Autodesk Inventor part; units mm, degrees
ref_plane "YZ Plane" through (0, 0, 0) normal (1, 0, 0) x (0, 1, 0)
ref_plane "XZ Plane" through (0, 0, 0) normal (0, 1, 0) x (-1, 0, 0)
ref_plane "XY Plane" through (0, 0, 0) normal (0, 0, 1) x (1, 0, 0)
sketch "Sketch1" plane through (0, 0, 0) normal (0, 0, 1) x (1, 0, 0)
  line L0 (0, 0) -> (93.5, 0)
  line L1 (93.5, 0) -> (93.5, 150)
  line L2 (93.5, 150) -> (0, 150)
  line L3 (0, 150) -> (0, 0)
  dimension "d0" = 93.5
  dimension "d1" = 150
sketch "Sketch2" plane through (0, 0, 0) normal (1, 0, 0) x (0, 1, 0)
  circle A0 centre (0, 0) radius 12.5
  circle A1 centre (0, 0) radius 8.5
  line L0 (-12.5, 0) -> (12.5, 0)
  line L1 (12.5, 0) -> (12.5, 12.5)
  line L2 (12.5, 12.5) -> (-12.5, 12.5)
  line L3 (-12.5, 12.5) -> (-12.5, 0)
  circle A2 centre (150, 0) radius 12.5
  circle A3 centre (150, 0) radius 8.5
  line L4 (137.5, 0) -> (162.5, 0)
  line L5 (162.5, 0) -> (162.5, 12.5)
  line L6 (162.5, 12.5) -> (137.5, 12.5)
  line L7 (137.5, 12.5) -> (137.5, 0)
  line L8 (-12.5, 12.5) -> (-17.5, 12.5)
  line L9 (-17.5, 12.5) -> (-17.5, 0)
  line L10 (-17.5, 0) -> (-12.5, 0)
  line L11 (-12.5, 0) -> (-12.5, 12.5)
  line L12 (12.5, 12.5) -> (17.5, 12.5)
  line L13 (17.5, 12.5) -> (17.5, 0)
  line L14 (17.5, 0) -> (12.5, 0)
  line L15 (12.5, 0) -> (12.5, 12.5)
  point P0 (8.5, 0)
  point P1 (-8.5, 0)
  point P2 (150, 0)
  point P3 (12.5, 0)
  dimension "d2" = 25
  dimension "d3" = 17
  dimension "d6" = 5
  dimension "d7" = 5
  dimension "d8" = 35
extrude "Extrusion1" add sketch "Sketch2" along normal up to surface (93.5 mm away) contours L3 L2 A0 | A0 L0 A1 | L10 L9 L8 L3 | A0 L2 L1 | L1 L12 L13 L14 | A1 L0 picked at (11.0622, 0.9272) picked at (2.1208, 1.8788)
ref_plane "Work Plane1" through (46.75, 0, 0) normal (-1, 0, 0) x (0, 0, 1)
sketch "Sketch3" plane through (0, -17.5, 0) normal (0, -1, 0) x (1, 0, 0)
  line L0 (0, 12.5) -> (93.5, 12.5)
  line L1 (76, 12.5) -> (111, 12.5)
  line L2 (111, 12.5) -> (111, 0)
  line L3 (111, 0) -> (76, 0)
  line L4 (76, 0) -> (76, 12.5)
  line L5 (93.5, 12.5) -> (93.5, 0)
  circle A0 centre (93.5, 0) radius 8.5
  point P0 (0, 0)
  point P1 (93.5, 12.5)
  point P2 (102, 0)
  point P3 (85, 0)
  dimension "d9" = 35
  dimension "d33" = 17
extrude "Extrusion2" add sketch "Sketch3" against normal blind 55 contours L0 L5 A0 L3 L4 | L1 L2 L3 A0 L5 | A0 L3 L5 | L5 L3 A0
extrude "Extrusion4" cut sketch "Sketch3" along normal through all both and the other way through all contours A0 L3 L5 | L5 L3 A0
extrude "Extrusion3" cut sketch "Sketch2" along normal up to surface (93.5 mm away) contours A1 L0 picked at (2.1208, 1.8788)
mirror "Mirror1" about plane through (46.75, 0, 0) normal (-1, 0, 0) of "Extrusion2", "Extrusion4", "Extrusion3"
sketch "Sketch4" plane through (76, 17.5, 12.5) normal (0, 0, 1) x (1, 0, 0)
  line L0 (-93.5, -35) -> (35, -35)
  line L1 (0, 20) -> (35, 20)
  line L2 (0, 0) -> (0, 20)
  line L3 (-58.5, 0) -> (0, 0)
  line L4 (-58.5, 0) -> (-58.5, 20)
  line L5 (-58.5, 20) -> (-93.5, 20)
  line L6 (35, -35) -> (35, 20)
  line L7 (-93.5, -35) -> (-93.5, 20)
  point P0 (-76, -17.5)
extrude "Extrusion5" add sketch "Sketch4" along normal blind 5
sketch "Sketch5" plane through (76, 17.5, 0) normal (0, 0, -1) x (-1, 0, 0)
  circle A0 centre (-2.75, -2.75) radius 2
  line L0 (-9, -9) -> (67.5, -9)
  line L1 (-9, 20) -> (-9, -9)
  circle A1 centre (61.25, -2.75) radius 2
  circle A2 centre (-2.75, -32.25) radius 2
  circle A3 centre (61.25, -32.25) radius 2
  line L2 (67.5, -35) -> (67.5, -26)
  line L3 (67.5, -26) -> (-9, -26)
  point P0 (76, -17.5)
  dimension "d18" = 4
  dimension "d19" = 6.25
  dimension "d20" = 6.25
  dimension "d23" = 64
  dimension "d26" = 29.5
  dimension "d29" = 6.25
  dimension "d30" = 6.25
extrude "Extrusion6" cut sketch "Sketch5" against normal blind 10
equation "\"d7\" = d6"
equation "\"d9\" = d8"
equation "\"d33\" = d3"
properties part number "ElectronicsHalf"
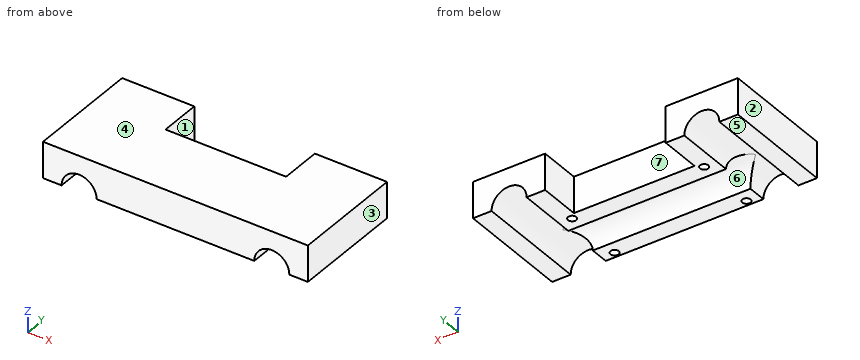
The model under review builds one solid part; all positions refer to its coordinate system, in mm. Face numbers are marked on the shaded views. A direction names the side the tool comes from. Round coordinates to 2 decimals unless told otherwise and drop trailing zeros. Loops run counter-clockwise (first coordinate to the right, second up) from the corner with the lowest first, then second, coordinate; pieces in that order, holes last. Notation, with made-up numbers: (33, 1.25) -> (54, 1.25) arc R20 ccw to (54, 28.25) -> close; hole circle Ø1 at (75, 65). An arc over 180 degrees is marked (long way). One line per question, with ' | ' between items. Start each with the question number.
Item 1: For pin 1 (3.5 mm diameter, centred on x = 78.75, y = 14.75, fed in from -Z); pin 2 (4 mm diameter, centred on x = 48.5, z = 10, fed in from +Y), all flat-tipped, find the tip position at first contact; note any pin that passes through.
Item 2: Add section D-D, the plane y = -14.75. Write out the cut boundary in (x, z), then the cut area to 3 significant figures.
Item 3: Add section C-C, the plane y = 10.5. Write out the cut boundary in (x, z), then the cut area to 3 significant figures.
Item 4: Add section B-B, the plane x = 78.75. Write out the cut boundary in (y, z), then the cut area to 3 significant figures.
Item 5: Wall thickness on line 1 along X through (y, z) = (32, 16); line 2 along Y through (x, z) = (14.75, 2.25); line 3 along Y through (x, z) = (78.75, 7.75): over which ranges is each line inside the solid? List them lowest first. Write a range as [from, to].
Item 6: Machinability: for the marked faces 5, 6 and 7, which of the approach directions +Z, -Z, +X, -X, +Y, -Y give a long, thin tool a straight path to every point of the face, cutting with its end or side? Answer none if there is none.
Item 7: Add section A-A, the plane z = 15.5. Write out the cut boundary in (x, y).
Item 8: Draft analysis for pull direction X (two halves, no side actions). For the marked faces 1, 2, 3 and 4, state which applies: +X half, -X half, draft (parallel to the pull), parting line (faces both ways), or undercut.
Return value:
1) pin 1: stops at z = 10 | pin 2: stops at y = 17.5
2) outline: (-17.5, 0) -> (-8.5, 0) arc R8.5 cw to (8.5, 0) -> (12.75, 0) -> (12.75, 10) -> (16.75, 10) -> (16.75, 0) -> (76.75, 0) -> (76.75, 10) -> (80.75, 10) -> (80.75, 0) -> (85, 0) arc R8.5 cw to (102, 0) -> (111, 0) -> (111, 17.5) -> (-17.5, 17.5) -> close | area: 1,940 mm2
3) outline: (-17.5, 0) -> (-8.5, 0) arc R8.5 cw to (8.5, 0) -> (85, 0) arc R8.5 cw to (102, 0) -> (111, 0) -> (111, 17.5) -> (-17.5, 17.5) -> close | area: 2,020 mm2
4) outline: (-17.5, 0) -> (-16.75, 0) -> (-16.75, 10) -> (-12.75, 10) -> (-12.75, 0) -> (-8.5, 0) arc R8.5 cw to (8.5, 0) -> (12.75, 0) -> (12.75, 10) -> (16.75, 10) -> (16.75, 0) -> (37.5, 0) -> (37.5, 17.5) -> (-17.5, 17.5) -> close | area: 769 mm2
5) line 1: x = [-17.5, 17.5], [76, 111] | line 2: y = [-17.5, -16.75], [-12.75, -8.2], [8.2, 12.75], [16.75, 37.5] | line 3: y = [-17.5, -16.75], [-12.75, -3.49], [3.49, 12.75], [16.75, 37.5]
6) face 5: -Z, +X, -X, +Y, -Y | face 6: -Z | face 7: +Z, -Z, +Y
7) outline: (-17.5, -17.5) -> (111, -17.5) -> (111, 37.5) -> (76, 37.5) -> (76, 17.5) -> (17.5, 17.5) -> (17.5, 37.5) -> (-17.5, 37.5) -> close
8) face 1: undercut | face 2: -X half | face 3: +X half | face 4: draft
